from build123d import *

# Parameters (mm, degrees)
F0_W     = 20
F0_H     = 6
F1_DEPTH = 37
F2_W     = 13.574068
F2_H     = 22.032887
F2_W_2   = 8.901329
F2_H_2   = 8.866575
F3_DEPTH = 12.5
F4_W     = 22.673105
F4_H     = 28.148874
F5_DEPTH = 12.5


with BuildPart() as f1:
    # F0 (on Top) → F1 (new body)
    with BuildSketch(Plane.XY):
        with Locations((0.443081, 0)):
            Rectangle(F0_W, F0_H)
        Polygon((-9.556919, 3), (10.443081, 3), (-9.556919, 5.455691), align=None)
    extrude(amount=F1_DEPTH)

    # F2 (on Right) → F3 (cut, symmetric)
    with BuildSketch(Plane.YZ):
        with Locations((5.025405, 13.710695)):
            Rectangle(F2_W, F2_H)
        with Locations((-1.928942, 30.943508)):
            Rectangle(F2_W_2, F2_H_2)
    extrude(amount=F3_DEPTH, both=True, mode=Mode.SUBTRACT)

    # F4 (on Front) → F5 (cut, symmetric)
    with BuildSketch(Plane.XZ):
        with Locations((9.403651, 19.088611)):
            Rectangle(F4_W, F4_H)
    extrude(amount=F5_DEPTH, both=True, mode=Mode.SUBTRACT)


solid = f1.part
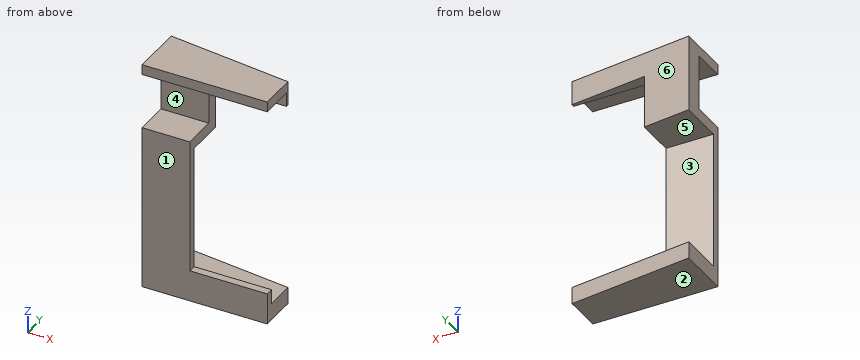
Could you check a few things on this model? Use its own coordinates, in mm. Face numbers are marked on the shaded views. A direction names the side the tool comes from. Give positions to 0.01 mm unless a question says otherwise; leave off trailing zeros. Order: outer loops, then holes, each group sorted by start corner. A loop starts at its lowest first (then second) coordinate and runs counter-clockwise, first axis right, second up.
1. Suppose I cut it at C-C (z = 23). Write out the boundary of the cut face in (x, y), plus the area to 3 significant figures.
Answers below:
outline: (-9.56, -3) - (-1.93, -3) - (-1.93, -1.76) - (-9.56, -1.76) - close
area: 9.44 mm2
2. Suppose I cut it at A-A (y = -0.25). Write out the boundary of the cut face in (x, z), plus the area to 3 significant figures.
Answers below:
outline: (-9.56, 0) - (10.44, 0) - (10.44, 2.69) - (-9.56, 2.69) - close; (-9.56, 24.73) - (-1.93, 24.73) - (-1.93, 26.51) - (-9.56, 26.51) - close; (-9.56, 35.38) - (10.44, 35.38) - (10.44, 37) - (-9.56, 37) - close
area: 99.9 mm2
3. Suppose I cut it at D-D (x = -5.5). Write out the boundary of the cut face in (y, z).
Answers below:
outline: (-3, 0) - (4.96, 0) - (4.96, 2.69) - (-1.76, 2.69) - (-1.76, 24.73) - (4.96, 24.73) - (4.96, 37) - (-3, 37) - (-3, 35.38) - (2.52, 35.38) - (2.52, 26.51) - (-3, 26.51) - close
4. For pin 1 (4.5 mm diameter, centred on x = -3.5, y = -1, fed in from -Z); pin 2 (4 mm diameter, centred on y = -1, z = 20.5, fed in from +X); pin 3 (4.5 mm diameter, centred on x = 3.5, z = 31, fed in from -Y), each with a flat end and sliding along its axis, tell me the tip position at first contact or that it passes through.
Answers below:
pin 1: stops at z = 0
pin 2: stops at x = -1.93
pin 3: stops at y = 2.52
5. Which directions (+Z, -Z, +X, -X, +Y, -Y) give clear straight access to the entire face, cutting with the end or side of a thin tool? Please do the marked faces 4, 5 and 6.
Answers below:
face 4: +X, -X, -Y
face 5: +X, -X, +Y
face 6: +Z, -Z, +X, +Y
6. I need wall thicknesses on L1, parallel to Z at x = -2.75, y = -1.25; L2, parallel to Z at x = -4, y = -2; L3, parallel to Z at x = 0.75, y = -1.25. Which ranges of each line are inside material? Lowest first, please.
Answers below:
L1: z = 0 to 2.69, 24.73 to 26.51, 35.38 to 37
L2: z = 0 to 26.51, 35.38 to 37
L3: z = 0 to 2.69, 35.38 to 37
7. Thinking about a two-plate mould opening in Z: for the marked faces 1, 2 and 3, which applies, +Z half, -Z half, draft (parallel to the pull), parting line (faces both ways), or undercut?
Answers below:
face 1: draft
face 2: -Z half
face 3: undercut
8. Suppose I cut it at B-B (x = 5). Write out the boundary of the cut face in (y, z), plus the area to 3 significant figures.
Answers below:
outline: (-3, 0) - (3.67, 0) - (3.67, 2.69) - (-1.76, 2.69) - (-1.76, 5.01) - (-3, 5.01) - close; (-3, 35.38) - (2.52, 35.38) - (2.52, 33.16) - (3.67, 33.16) - (3.67, 37) - (-3, 37) - close
area: 34.2 mm2
